from build123d import *

# Parameters (mm, degrees)
BOX007_W     = 2.4
BOX007_H     = 24
BOX007_DEPTH = 30
BOX008_W     = 2.4
BOX008_H     = 24
BOX008_DEPTH = 30
BOX009_W     = 2.4
BOX009_H     = 24
BOX009_DEPTH = 30
BOX_W        = 2.4
BOX_H        = 24
BOX_DEPTH    = 30
BOX004_W     = 33
BOX004_H     = 30
BOX004_DEPTH = 22


with BuildPart() as box007:
    # Box007 → Box007 (new body)
    with BuildSketch(Plane(origin=(11.3, 3, 0), x_dir=(1, 0, 0), z_dir=(0, 0, 1))):
        with Locations((1.2, 12)):
            Rectangle(BOX007_W, BOX007_H)
    extrude(amount=BOX007_DEPTH)


with BuildPart() as box008:
    # Box008 → Box008 (new body)
    with BuildSketch(Plane(origin=(19.3, 3, 0), x_dir=(1, 0, 0), z_dir=(0, 0, 1))):
        with Locations((1.2, 12)):
            Rectangle(BOX008_W, BOX008_H)
    extrude(amount=BOX008_DEPTH)


with BuildPart() as box009:
    # Box009 → Box009 (new body)
    with BuildSketch(Plane(origin=(27.3, 3, 0), x_dir=(1, 0, 0), z_dir=(0, 0, 1))):
        with Locations((1.2, 12)):
            Rectangle(BOX009_W, BOX009_H)
    extrude(amount=BOX009_DEPTH)


with BuildPart() as fusion:
    # Box → Box (new body)
    with BuildSketch(Plane(origin=(3.3, 3, 0), x_dir=(1, 0, 0), z_dir=(0, 0, 1))):
        with Locations((1.2, 12)):
            Rectangle(BOX_W, BOX_H)
    extrude(amount=BOX_DEPTH)

    # Fusion: union Box007, Box008, Box009
    add(box007.part)
    add(box008.part)
    add(box009.part)


with BuildPart() as fusion_1:
    # Fusion placement: moved
    add(fusion.part.moved(Location((0, 0, 3))))


with BuildPart() as cut:
    # Box004 → Box004 (new body)
    with BuildSketch(Plane.XY):
        with Locations((16.5, 15)):
            Rectangle(BOX004_W, BOX004_H)
    extrude(amount=BOX004_DEPTH)

    # Cut: cut Fusion
    add(fusion_1.part, mode=Mode.SUBTRACT)


solid = cut.part
Check sheet for the modelled part. Datum: model origin and axes. Units: mm. A direction names the side the tool comes from. Coordinates: 2 decimals unless noted, no trailing zeros. Loops run counter-clockwise (first coordinate to the right, second up) from the corner with the lowest first, then second, coordinate; pieces in that order, holes last. Notation, with made-up numbers: (-16.75, 31) -> (0.25, 31) arc R16 cw to (0.25, 55) -> close; hole circle Ø9 at (8, 62). An arc over 180 degrees is marked (long way). Write item = value, one per line. Start each with the question number.
1. Material ranges on line 1 (X direction, y = 21.5, z = 6); line 2 (Y direction, x = 27.5, z = 3.75); line 3 (Z direction, x = 20, y = 10.5), recorded low to high.
2. Depth check by flat-ended pin: P1, Ø1.2, axis at x = 28.5, y = 14, coming from the +Z side; P2, Ø1, axis at x = 22.5, z = 5, coming from the -Y side. Enter the tip coordinate at first touch or a pass-through.
3. Tool access check on faces 1 (the flat face through (16, 15, 0)), 2 (the flat face through (4, 3, 12)). Record the directions out of +Z, -Z, +X, -X, +Y, -Y that give a thin tool (end or side, any length) a straight path to the whole face; none if there is none.
4. Section check C-C on x = 12. Record the cut outline in (y, z), then the cut area to 3 significant figures.
5. Section check A-A on z = 19. Record the cut outline in (x, y).
6. Draft check along Y on faces 3 (the flat face through (16, 15, 22)), 4 (the flat face through (16, 30, 11)), 5 (the flat face through (13.7, 15, 12)). Enter one of: released by +Y, released by -Y, zero draft, split by the parting line, or undercut.
7. Section check B-B on y = 10. Record the cut outline in (x, z).
Responses:
q1.line_1 = 0 to 3.3, 5.7 to 11.3, 13.7 to 19.3, 21.7 to 27.3, 29.7 to 33
q1.line_2 = 0 to 3, 27 to 30
q1.line_3 = 0 to 3
q2.P1 = 3
q2.P2 = 0
q3.face_1 = -Z, +X, -X, +Y, -Y
q3.face_2 = +Z
q4.outline = (0, 0) -> (30, 0) -> (30, 22) -> (27, 22) -> (27, 3) -> (3, 3) -> (3, 22) -> (0, 22) -> close
q4.area = 204 mm2
q5.outline = (0, 0) -> (33, 0) -> (33, 30) -> (0, 30) -> close; hole (3.3, 3) -> (5.7, 3) -> (5.7, 27) -> (3.3, 27) -> close; hole (11.3, 3) -> (13.7, 3) -> (13.7, 27) -> (11.3, 27) -> close; hole (19.3, 3) -> (21.7, 3) -> (21.7, 27) -> (19.3, 27) -> close; hole (27.3, 3) -> (29.7, 3) -> (29.7, 27) -> (27.3, 27) -> close
q6.face_3 = zero draft
q6.face_4 = released by +Y
q6.face_5 = undercut
q7.outline = (0, 0) -> (33, 0) -> (33, 22) -> (29.7, 22) -> (29.7, 3) -> (27.3, 3) -> (27.3, 22) -> (21.7, 22) -> (21.7, 3) -> (19.3, 3) -> (19.3, 22) -> (13.7, 22) -> (13.7, 3) -> (11.3, 3) -> (11.3, 22) -> (5.7, 22) -> (5.7, 3) -> (3.3, 3) -> (3.3, 22) -> (0, 22) -> close
